```python
from build123d import *

# Parameters (mm, degrees)
SALIENTE_EXTRUIR1_DEPTH = 3


with BuildPart() as part:
    # Model → Saliente-Extruir1 (new body)
    with BuildSketch(Plane.XY):
        with BuildLine():
            Line((25.488716275, 56.424131461), (28.178792169, 56.424131461))
            ThreePointArc((28.178792169, 56.424131461), (29.940174662, 55.85261488), (31.030450954, 54.355819272))
            ThreePointArc((31.030450954, 54.355819272), (34.201179997, 48.563621322), (39.252486332, 44.310694794))
            ThreePointArc((39.252486332, 44.310694794), (44.045367232, 38.357656573), (44.338099173, 30.720596968))
            ThreePointArc((44.338099173, 30.720596968), (42.619326371, 18.377856), (44.338099173, 6.035115032))
            ThreePointArc((44.338099173, 6.035115032), (44.045367232, -1.601944573), (39.252486332, -7.554982794))
            ThreePointArc((39.252486332, -7.554982794), (34.201179997, -11.807909322), (31.030450954, -17.600107272))
            ThreePointArc((31.030450954, -17.600107272), (29.940174662, -19.09690288), (28.178792169, -19.668419461))
            Line((28.178792169, -19.668419461), (25.488716275, -19.668419461))
            Line((25.488716275, -19.668419461), (25.488716275, -9.668419461))
            Line((25.488716275, -9.668419461), (22.488716275, -9.668419461))
            Line((22.488716275, -9.668419461), (22.488716275, 0.331580539))
            Line((22.488716275, 0.331580539), (25.488716275, 0.331580539))
            Line((25.488716275, 0.331580539), (25.488716275, 36.424131461))
            Line((25.488716275, 36.424131461), (22.488716275, 36.424131461))
            Line((22.488716275, 36.424131461), (22.488716275, 46.424131461))
            Line((22.488716275, 46.424131461), (25.488716275, 46.424131461))
            Line((25.488716275, 46.424131461), (25.488716275, 56.424131461))
        make_face()
    extrude(amount=SALIENTE_EXTRUIR1_DEPTH)


solid = part.part
```
Model file for the job. Use its own axes, mm. A direction names the side the tool comes from. Give positions to 0.01 mm unless a question says otherwise; leave off trailing zeros. Loops run counter-clockwise (first coordinate to the right, second up) from the corner with the lowest first, then second, coordinate; pieces in that order, holes last. Notation, with made-up numbers: (17.5, 43) - (36.5, 43) arc R24 ccw to (36.5, 54) - close; hole circle Ø10 at (-39.75, 49.5). An arc over 180 degrees is marked (long way). One line per item, written item: value. Start each with the question number.
1. Probe L1, parallel to X at y = 17.5, z = 1; L2, parallel to X at y = 25.5, z = 0.25; L3, parallel to Y at x = 31.5, z = 2.2. List the from-to ranges inside material, lowest first. Write a range as from..to.
2. Pin check, flat tips, straight feed: pin 1 (3 mm diameter, centred on x = 36, y = 11, fed in from -Z); pin 2 (1 mm diameter, centred on x = 35.5, z = 2, fed in from -Y); pin 3 (1.5 mm diameter, centred on x = 23.5, z = 1, fed in from +Y); pin 4 (1.5 mm diameter, centred on x = 24, z = 2, fed in from -Y). Stop position of each tip, or through.
3. Slice it at A-A (z = 1.55). List the corners of the cut face in (x, y).
4. Slice it at C-C (x = 41.25). List the corners of the cut face in (y, z).
5. Slice it at B-B (y = 7). List the corners of the cut face in (x, z).
6. Which spindle directions (+Z, -Z, +X, -X, +Y, -Y) get a long thin tool onto all of the face, cutting with end or side? Do faces 1 (the flat face through (24, 0.332, 1)), 2 (the flat face through (24, -9.668, 1)), 3 (the flat face through (25.489, 51, 1)). Say none if no direction does.
7. Pull direction Y, two halves, no side cores. Call faces 4 (the flat face through (34, 19, 3)), 5 (the flat face through (24, 46.424, 1)), 6 (the flat face through (24, 36.424, 1)), 7 (the cylindrical face through (29.96, -19.08, 1.48)): pulls with the +Y half, pulls with the -Y half, needs draft (parallel to the pull), parting line crosses it, or undercut.
Solution:
1. L1: x = 25.49..42.63
1. L2: x = 25.49..43.18
1. L3: y = -16.33..53.08
2. pin 1: stops at z = 0
2. pin 2: stops at y = -10.9
2. pin 3: stops at y = 46.42
2. pin 4: stops at y = -9.67
3. outline: (22.49, -9.67) - (25.49, -9.67) - (25.49, -19.67) - (28.18, -19.67) arc R3 ccw to (31.03, -17.6) arc R17.94 cw to (39.25, -7.55) arc R12.16 ccw to (44.34, 6.04) arc R45.18 cw to (44.34, 30.72) arc R12.16 ccw to (39.25, 44.31) arc R17.94 cw to (31.03, 54.36) arc R3 ccw to (28.18, 56.42) - (25.49, 56.42) - (25.49, 46.42) - (22.49, 46.42) - (22.49, 36.42) - (25.49, 36.42) - (25.49, 0.33) - (22.49, 0.33) - close
4. outline: (-5.94, 0) - (42.7, 0) - (42.7, 3) - (-5.94, 3) - close
5. outline: (25.49, 0) - (44.08, 0) - (44.08, 3) - (25.49, 3) - close
6. face 1: +Z, -Z, -X
6. face 2: +Z, -Z, -X, -Y
6. face 3: +Z, -Z, -X, +Y
7. face 4: needs draft
7. face 5: pulls with the +Y half
7. face 6: undercut
7. face 7: pulls with the -Y half
